from build123d import *

# Parameters (mm, degrees)
BOSS_EXTRUDE1_DEPTH = 200
SKETCH2_W           = 34
SKETCH2_H           = 135
SKETCH2_W_2         = 26
SKETCH2_H_2         = 65
SKETCH2_W_3         = 27.5
SKETCH2_W_4         = 31.5
SKETCH2_H_3         = 33
CUT_EXTRUDE1_DEPTH  = 200
SKETCH3_W           = 32.5
SKETCH3_H           = 30
BOSS_EXTRUDE2_DEPTH = 9.25
FILLET1_R           = 10


with BuildPart() as part:
    # Sketch1 → Boss-Extrude1 (new body)
    with BuildSketch(Plane(origin=(0, 0, 0), x_dir=(1, 0, 0), z_dir=(0, 1, 0))):
        Polygon((-38, -10.75), (-45.5, -10.75), (-45.5, 19.25), (53, 19.25), (73.75, -13.25), (137.04, -13.25), (137.04, -22.5), (257.04, -22.5), (257.04, -34.25), (43, -34.25), (43, 10.75), (-38, 10.75), align=None)
    extrude(amount=BOSS_EXTRUDE1_DEPTH)

    # Sketch2 → Cut-Extrude1 (cut)
    with BuildSketch(Plane(origin=(0, 0, 13.25), x_dir=(-1, 0, 0), z_dir=(0, 0, -1))):
        with Locations((-117.75, 121.5)):
            Rectangle(SKETCH2_W, SKETCH2_H)
        with Locations((-212.54, 164.5)):
            Rectangle(SKETCH2_W_2, SKETCH2_H_2)
        with Locations((-212.54, 70.5)):
            Rectangle(SKETCH2_W_2, SKETCH2_H_2)
        with Locations((-184.79, 119.5)):
            Rectangle(SKETCH2_W_3, SKETCH2_H_2)
        with Locations((-153.79, 46.5)):
            Rectangle(SKETCH2_W_4, SKETCH2_H_3)
    extrude(amount=-CUT_EXTRUDE1_DEPTH, mode=Mode.SUBTRACT)

    # Sketch3 → Boss-Extrude2 (add)
    with BuildSketch(Plane(origin=(0, 0, 22.5), x_dir=(-1, 0, 0), z_dir=(0, 0, -1))):
        with Locations((-153.29, 15)):
            Rectangle(SKETCH3_W, SKETCH3_H)
    extrude(amount=BOSS_EXTRUDE2_DEPTH)

    # Fillet1
    fillet1_edges = [part.edges().sort_by_distance(p)[0] for p in [
        (257.04, 0, 28.375),
        (257.04, 200, 28.375),
        (53, 100, -19.25),
        (73.75, 100, 13.25),
    ]]
    fillet(fillet1_edges, radius=FILLET1_R)


solid = part.part
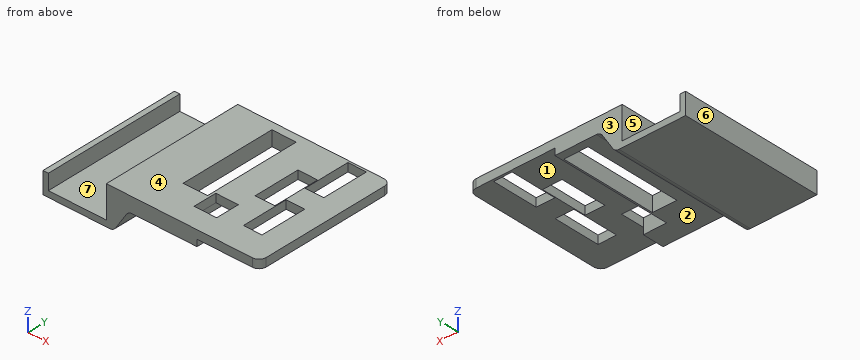
CAD build for the part. Positions are in the model's coordinates, mm. Face numbers are marked on the shaded views. A direction names the side the tool comes from. Coordinates: 2 decimals unless noted, no trailing zeros. Order: outer loops, then holes, each group sorted by start corner. A loop starts at its lowest first (then second) coordinate and runs counter-clockwise, first axis right, second up. Notation, with made-up numbers: (41.25, -35.75) -> (83.25, -35.75) arc R18 cw to (83.25, -24.75) -> close; hole circle Ø9 at (56.5, -7.5). An arc over 180 degrees is marked (long way). Answer in a Markdown table with one row per item.
1) Band-saw the part on C-C (z = 25.5). List the corners of the cut face in (x, y), and give its area (3 significant figures).
Check values:
| item | result |
|---|---|
| outline | (43, 0) -> (247.04, 0) arc R10 ccw to (257.04, 10) -> (257.04, 190) arc R10 ccw to (247.04, 200) -> (43, 200) -> close; hole (100.75, 54) -> (134.75, 54) -> (134.75, 189) -> (100.75, 189) -> close; hole (138.04, 30) -> (169.54, 30) -> (169.54, 63) -> (138.04, 63) -> close; hole (171.04, 87) -> (198.54, 87) -> (198.54, 152) -> (171.04, 152) -> close; hole (199.54, 38) -> (225.54, 38) -> (225.54, 103) -> (199.54, 103) -> close; hole (199.54, 132) -> (225.54, 132) -> (225.54, 197) -> (199.54, 197) -> close |
| area | 32,000 mm2 |
2) Flat gauge pins, fed straight in: P1, Ø7.5, axis at y = 91.5, z = 16.5, coming from the +X side; P2, Ø8, axis at y = 110.5, z = -12, coming from the +X side; P3, Ø4, axis at x = 222, y = 153.5, coming from the -Z side; P4, Ø9.5, axis at y = 43, z = 26.5, coming from the -X side. Where does each tip first touch, or does it go through?
Check values:
| item | result |
|---|---|
| P1 | x = 137.04 |
| P2 | x = 60.18 |
| P3 | through |
| P4 | x = 43 |
3) Band-saw the part on D-D (x = 131.5). List the corners of the cut face in (y, z), and give its area (4 significant figures).
Check values:
| item | result |
|---|---|
| outline | (0, 13.25) -> (54, 13.25) -> (54, 34.25) -> (0, 34.25) -> close; (189, 13.25) -> (200, 13.25) -> (200, 34.25) -> (189, 34.25) -> close |
| area | 1,365 mm2 |
4) Mould opens along X. For the marked faces 4, 5, 6 and 7 say: pulls with the +X half, pulls with the -X half, needs draft (parallel to the pull), parting line crosses it, or undercut.
Check values:
| item | result |
|---|---|
| face 4 | needs draft |
| face 5 | undercut |
| face 6 | pulls with the -X half |
| face 7 | undercut |
5) Drill centre lines: line 1 (X direction, y = 98, z = 23.5); line 2 (X direction, y = 111, z = 23.5); line 3 (X direction, y = 155.5, z = 14). Where is each one in solid material? Low to high.
Check values:
| item | result |
|---|---|
| line 1 | 43 to 100.75, 134.75 to 171.04, 198.54 to 199.54, 225.54 to 257.04 |
| line 2 | 43 to 100.75, 134.75 to 171.04, 198.54 to 257.04 |
| line 3 | 43 to 100.75, 134.75 to 137.04 |
6) Band-saw the part on B-B (x = 218). List the corners of the cut face in (y, z).
Check values:
| item | result |
|---|---|
| outline | (0, 22.5) -> (38, 22.5) -> (38, 34.25) -> (0, 34.25) -> close; (103, 22.5) -> (132, 22.5) -> (132, 34.25) -> (103, 34.25) -> close; (197, 22.5) -> (200, 22.5) -> (200, 34.25) -> (197, 34.25) -> close |
7) Which spindle directions (+Z, -Z, +X, -X, +Y, -Y) get a long thin tool onto all of the face, cutting with end or side? Do the marked faces 1, 2 and 3. Say none if no direction does.
Check values:
| item | result |
|---|---|
| face 1 | -Z, +X, +Y |
| face 2 | -Z, +X, +Y, -Y |
| face 3 | +Z, -Z, +X, -X, +Y |
8) Band-saw the part on A-A (y = 78.5). List the corners of the cut face in (x, z), and give its area (3 significant figures).
Check values:
| item | result |
|---|---|
| outline | (-45.5, -19.25) -> (47.52, -19.25) arc R10 ccw to (55.95, -14.63) -> (70.8, 8.63) arc R10 cw to (79.23, 13.25) -> (100.75, 13.25) -> (100.75, 34.25) -> (43, 34.25) -> (43, -10.75) -> (-38, -10.75) -> (-38, 10.75) -> (-45.5, 10.75) -> close; (134.75, 13.25) -> (137.04, 13.25) -> (137.04, 22.5) -> (199.54, 22.5) -> (199.54, 34.25) -> (134.75, 34.25) -> close; (225.54, 22.5) -> (257.04, 22.5) -> (257.04, 34.25) -> (225.54, 34.25) -> close |
| area | 3,940 mm2 |
